Check sheet for the modelled part. Datum: model origin and axes. Units: mm. Give positions to 0.01 mm unless a question says otherwise; leave off trailing zeros. Write each loop counter-clockwise with the first axis right and the second up, starting at its lowest first coordinate (ties: lowest second). Pieces come first, ordered by that corner, then holes. Notation, with made-up numbers: (32, 8) -> (59, 8) arc R31 cw to (59, 41) -> close; hole circle Ø5 at (27, 79.5). An arc over 180 degrees is marked (long way). Return JSON: item names as keys, results as strings.
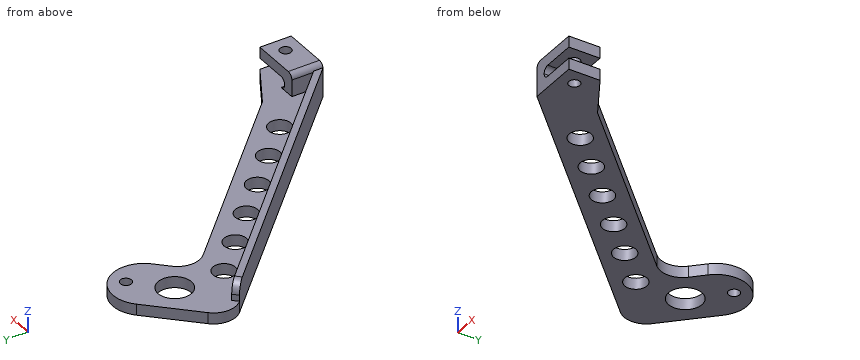
from build123d import *

# Parameters (mm, degrees)
F0_R     = 5
F0_R_2   = 7.5
F0_R_3   = 2.5
F1_DEPTH = 5
F3_DEPTH = 14
F5_R     = 2.5
F6_DEPTH = 25
F7_R     = 2.5
F8_DEPTH = 5
F4_W     = 150
F4_H     = 5
F9_DEPTH = 3


with BuildPart() as f1:
    # F0 (on Top) → F1 (new body)
    with BuildSketch(Plane.XY):
        with BuildLine():
            Line((15, 7), (-4.0848081724, 18.2269437961))
            Line((-4.0848081724, 18.2269437961), (-79.2670273048, 93.4091629285))
            ThreePointArc((-79.2670273048, 93.4091629285), (-82.1959594929, 100.4802307404), (-79.2670273048, 107.5512985522))
            Line((-79.2670273048, 107.5512985522), (-73.8864699203, 112.9318559367))
            ThreePointArc((-73.8864699203, 112.9318559367), (-73.8864699203, 132.7308458099), (-93.6854597935, 132.7308458099))
            Line((-93.6854597935, 132.7308458099), (-113.2081528017, 113.2081528017))
            ThreePointArc((-113.2081528017, 113.2081528017), (-116.1370849898, 106.1370849898), (-113.2081528017, 99.066017178))
            Line((-113.2081528017, 99.066017178), (-7.1421356237, -7))
            Line((-7.1421356237, -7), (15, -7))
            Line((15, -7), (15, 7))
        make_face()
        with Locations((-64.4147610714, 64.4208090516)):
            Circle(F0_R, mode=Mode.SUBTRACT)
        with Locations((-21.9838184576, 21.998938408)):
            Circle(F0_R, mode=Mode.SUBTRACT)
        with Locations((-36.1274659955, 36.1395619558)):
            Circle(F0_R, mode=Mode.SUBTRACT)
        with Locations((-50.2711135335, 50.2801855037)):
            Circle(F0_R, mode=Mode.SUBTRACT)
        with Locations((-92.7020561473, 92.7020561473)):
            Circle(F0_R, mode=Mode.SUBTRACT)
        with Locations((-78.5584086094, 78.5614325994)):
            Circle(F0_R, mode=Mode.SUBTRACT)
        with Locations((-92.1330977986, 114.4842179316)):
            Circle(F0_R_2, mode=Mode.SUBTRACT)
        with Locations((-78.8362173886, 127.7810983416)):
            Circle(F0_R_3, mode=Mode.SUBTRACT)
    extrude(amount=F1_DEPTH)


with BuildPart() as f3:
    # F2 (on face) → F3 (new body)
    with BuildSketch(Plane.XZ.offset(7)):
        with BuildLine():
            Line((-7.1421356237, 12.5), (-7.1421356237, 5))
            Line((-7.1421356237, 5), (0.3578643763, 5))
            ThreePointArc((0.3578643763, 5), (-1.4099025767, 5.732233047), (-2.1421356237, 7.5))
            ThreePointArc((-2.1421356237, 7.5), (-1.4099025767, 9.267766953), (0.3578643763, 10))
            Line((0.3578643763, 10), (15, 10))
            Line((15, 10), (15, 15))
            Line((15, 15), (-4.6421356237, 15))
            ThreePointArc((-4.6421356237, 15), (-6.4099025767, 14.267766953), (-7.1421356237, 12.5))
        make_face()
    extrude(amount=-F3_DEPTH)


with BuildPart() as f6_tool:
    # F5 (on face) → F6 (new body)
    with BuildSketch(Plane(origin=(0, 0, 0), x_dir=(1, 0, 0), z_dir=(0, 0, -1))):
        with Locations((8, 0)):
            Circle(F5_R)
    extrude(amount=-F6_DEPTH)


with BuildPart() as f1_1:
    add(f1.part)

    # F6: cut by f6_tool
    add(f6_tool.part, mode=Mode.SUBTRACT)

    # F7 (on face) → F8 (cut)
    with BuildSketch(Plane.XY.offset(15)):
        with Locations((8, 0)):
            Circle(F7_R)
    extrude(amount=-F8_DEPTH, mode=Mode.SUBTRACT)



with BuildPart() as f3_1:
    add(f3.part)

    # F6: cut by f6_tool
    add(f6_tool.part, mode=Mode.SUBTRACT)


with BuildPart() as f1_2:
    add(f1_1.part)

    add(f3_1.part)  # F9 merges F3
    # F4 (on face) → F9 (join)
    with BuildSketch(Plane(origin=(-7.0710678119, -7.0710678119, 0), x_dir=(0.7071067812, -0.7071067812, 0), z_dir=(-0.7071067812, -0.7071067812, 0))):
        with Locations((-75.1005050634, 2.5)):
            Rectangle(F4_W, F4_H)
        with BuildLine():
            Line((-150.1005050634, 5), (-0.1005050634, 5))
            Line((-0.1005050634, 5), (-0.1005050634, 13))
            Line((-0.1005050634, 13), (-145.1080126235, 12.782269238))
            ThreePointArc((-145.1080126235, 12.782269238), (-148.638692297, 11.3151534598), (-150.1005050634, 7.7822748743))
            Line((-150.1005050634, 7.7822748743), (-150.1005050634, 5))
        make_face()
    extrude(amount=-F9_DEPTH)


solid = f1_2.part
(1) Cross-section at C-C on z = 2. State how many separate pieces and enclosed holes the cut face has, then the cut area to 3 significant figures.
Reply:
{"separate pieces": "1", "enclosed holes": "9", "area": "3,570 mm^2"}
(2) Cross-section at D-D on y = 117.5. Enter the section's corners in (x, z).
Reply:
{"outline": "(-108.92, 0) -> (-99, 0) -> (-99, 5) -> (-108.92, 5) -> close; (-85.27, 0) -> (-70.84, 0) -> (-70.84, 5) -> (-85.27, 5) -> close"}
(3) Depth check by flat-ended pin: pin 1 Ø4 at (y, z) = (84.5, 5.5) entering from +X; pin 2 Ø1.5 at (x, z) = (-45, 4) entering from +Y; pin 3 Ø10 at (x, y) = (-18, 14) entering from -Z; pin 4 Ø11.5 at (x, y) = (-50.27, 50.28) entering from +Z. Enter the tip coordinate at first touch or a pass-through.
Reply:
{"pin 1": "x = -68.42", "pin 2": "y = 59.89", "pin 3": "z = 0", "pin 4": "z = 5"}
(4) Cross-section at B-B on y = 0. Enter the section's corners in (x, z), then the cut area to 3 significant figures.
Reply:
{"outline": "(-14.14, 0) -> (5.5, 0) -> (5.5, 5) -> (0.36, 5) arc R2.5 cw to (0.36, 10) -> (5.5, 10) -> (5.5, 15) -> (-4.64, 15) arc R2.5 ccw to (-7.14, 12.5) -> (-7.14, 5) -> (-9.9, 5) -> (-9.9, 12.99) -> (-14.14, 12.99) -> close; (10.5, 0) -> (15, 0) -> (15, 5) -> (10.5, 5) -> close; (10.5, 10) -> (15, 10) -> (15, 15) -> (10.5, 15) -> close", "area": "267 mm^2"}
(5) Cross-section at A-A on x = 8. Enter the section's corners in (y, z).
Reply:
{"outline": "(-7, 0) -> (-2.5, 0) -> (-2.5, 5) -> (-7, 5) -> close; (-7, 10) -> (-2.5, 10) -> (-2.5, 15) -> (-7, 15) -> close; (2.5, 0) -> (11.12, 0) -> (11.12, 5) -> (2.5, 5) -> close; (2.5, 10) -> (7, 10) -> (7, 15) -> (2.5, 15) -> close"}
(6) Thickness scan on L1, parallel to Y at x = -78.5, z = 4.75; L2, parallel to Y at x = 8, z = 2; L3, parallel to X at y = 82, z = 2.25. Record the ranges inside material, lowest first.
Reply:
{"L1": "64.36 to 73.56, 83.56 to 92.64, 108.32 to 125.3, 130.26 to 135.8", "L2": "-7 to -2.5, 2.5 to 11.12", "L3": "-96.14 to -82.19, -74.93 to -67.86"}
